Design review of the part built by this model. Coordinates are the model's own, in mm. A direction names the side the tool comes from. Round coordinates to 2 decimals unless told otherwise and drop trailing zeros. Order: outer loops, then holes, each group sorted by start corner. A loop starts at its lowest first (then second) coordinate and runs counter-clockwise, first axis right, second up. Notation, with made-up numbers: (-23, -19) - (1, -19) arc R27 ccw to (1, 9) - close; hole circle Ø3 at (63, -6). An arc over 180 degrees is marked (long way). Answer as a JSON object with one key per item and string values. Group by question number.
from build123d import *

# Parameters (mm, degrees)
SKETCH1_W           = 147.32
SKETCH1_H           = 25.4
SKETCH1_R           = 1.4351
SKETCH1_W_2         = 25.4
SKETCH1_H_2         = 96.52
BOSS_EXTRUDE1_DEPTH = 6.35


with BuildPart() as part:
    # Sketch1 → Boss-Extrude1 (new body)
    with BuildSketch(Plane.XY):
        with Locations((0, 60.96)):
            Rectangle(SKETCH1_W, SKETCH1_H)
        with Locations((0, 51.6255)):
            Circle(SKETCH1_R, mode=Mode.SUBTRACT)
        with Locations((-60.96, 0)):
            Rectangle(SKETCH1_W_2, SKETCH1_H_2)
        with Locations((-51.6255, 0)):
            Circle(SKETCH1_R, mode=Mode.SUBTRACT)
        with Locations((60.96, 0)):
            Rectangle(SKETCH1_W_2, SKETCH1_H_2)
        with Locations((51.6255, 0)):
            Circle(SKETCH1_R, mode=Mode.SUBTRACT)
        Polygon((-48.26, -48.26), (-73.66, -48.26), (-73.66, -73.66), (73.66, -73.66), (73.66, -48.26), (48.26, -48.26), align=None)
        with Locations((0, -51.6255)):
            Circle(SKETCH1_R, mode=Mode.SUBTRACT)
    extrude(amount=BOSS_EXTRUDE1_DEPTH)


solid = part.part
1. Clearance check with a flat-ended pin moving along its axis: P1, Ø4.5, axis at x = 51.63, y = 0, coming from the -Z side. State where the tip first meets the part, or that it passes through.
2. Tool access review of faces 4 (the flat face through (-73.66, 1, 3)), 5 (the flat face through (1, -48.26, 3)): name each direction out of +Z, -Z, +X, -X, +Y, -Y from which nothing blocks a thin tool from reaching the whole face with its end or side.
3. Take a section at A-A, the plane y = 8. Give the boundary of the cut face in (x, z).
4. Mouldability with a two-part tool opening along Y and no side actions: class faces 1 (the flat face through (73.66, -1, 3)), 2 (the flat face through (48.26, -1, 3)), 3 (the flat face through (-1, -73.66, 3)) as pulls with the +Y half, pulls with the -Y half, needs draft (parallel to the pull), parting line crosses it, or undercut.
5. To check wall thickness, follow line 1 (Y direction, x = 0, z = 4.5); line 2 (X direction, y = 26, z = 6). State the ranges of each line that lie inside material, in increasing order. Write a range as from..to.
6. Take a section at C-C, the plane z = 1.5. Give the boundary of the cut face in (x, y).
Response values:
{
 "1": {"P1": "z = 0"},
 "2": {"face 4": "+Z, -Z, -X, +Y, -Y", "face 5": "+Z, -Z"},
 "3": {"outline": "(-73.66, 0) - (-48.26, 0) - (-48.26, 6.35) - (-73.66, 6.35) - close; (48.26, 0) - (73.66, 0) - (73.66, 6.35) - (48.26, 6.35) - close"},
 "4": {"face 1": "needs draft", "face 2": "undercut", "face 3": "pulls with the -Y half"},
 "5": {"line 1": "-73.66..-53.06, -50.19..-48.26, 48.26..50.19, 53.06..73.66", "line 2": "-73.66..-48.26, 48.26..73.66"},
 "6": {"outline": "(-73.66, -73.66) - (73.66, -73.66) - (73.66, 73.66) - (-73.66, 73.66) - close; hole circle Ø2.87 at (-51.63, 0); hole (-48.26, -48.26) - (48.26, -48.26) - (48.26, 48.26) - (-48.26, 48.26) - close; hole circle Ø2.87 at (0, -51.63); hole circle Ø2.87 at (0, 51.63); hole circle Ø2.87 at (51.63, 0)"}
}
